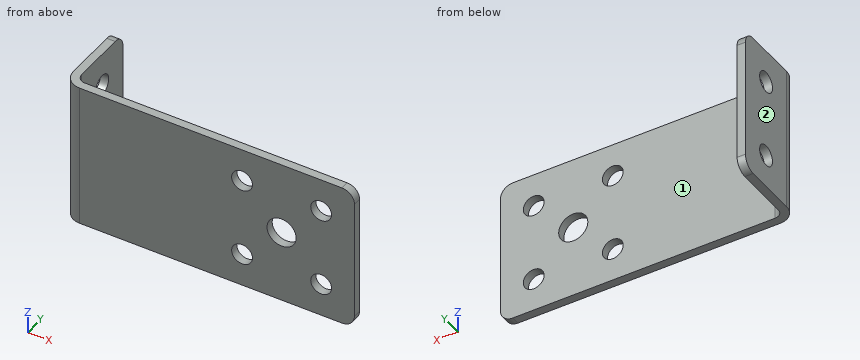
from build123d import *

# Parameters (mm, degrees)
SKETCH1_W                    = 70
SKETCH1_H                    = 35
BASE_FLANGE1_DEPTH           = 2
EDGE_FLANGE1_STRIP_W         = 12
EDGE_FLANGE1_STRIP_H         = 2
EDGE_FLANGE1_STRIP_CUT_DEPTH = 35
EDGE_FLANGE1_DEPTH           = 35
F_5_0MM_DOWEL_HOLE1_D        = 5
F_5_0MM_DOWEL_HOLE2_D        = 7
F_5_0MM_DOWEL_HOLE3_D        = 5
FILLET1_R                    = 3


# Sheet-metal steps are written as plain solids
with BuildPart() as part:
    # Sketch1 → Base-Flange1 (new body)
    with BuildSketch(Plane(origin=(0, 0, 0), x_dir=(1, 0, 0), z_dir=(0, 1, 0))):
        Rectangle(SKETCH1_W, SKETCH1_H)
    extrude(amount=BASE_FLANGE1_DEPTH)

    # Edge-Flange1 strip (across the edge) → Edge-Flange1 strip cut (cut)
    with BuildSketch(Plane(origin=(-35, 2, -17.5), x_dir=(1, 0, 0), z_dir=(0, 0, 1))):
        with Locations((-2, -1)):
            Rectangle(EDGE_FLANGE1_STRIP_W, EDGE_FLANGE1_STRIP_H)
    extrude(amount=EDGE_FLANGE1_STRIP_CUT_DEPTH, mode=Mode.SUBTRACT)

    # Edge-Flange1 section (across the edge) → Edge-Flange1 (add)
    with BuildSketch(Plane(origin=(-35, 2, -17.5), x_dir=(1, 0, 0), z_dir=(0, 0, 1))):
        with BuildLine():
            Line((0, 2), (0, 18))
            Line((0, 18), (2, 18))
            Line((2, 18), (2, 2))
            ThreePointArc((2, 2), (2.585786438, 0.585786438), (4, 0))
            Line((4, 0), (4, -2))
            ThreePointArc((4, -2), (1.171572875, -0.828427125), (0, 2))
        make_face()
    extrude(amount=EDGE_FLANGE1_DEPTH)

    # Ø5.0mm Dowel Hole1 (through all)
    with Locations(Plane(origin=(0, 2, 0), x_dir=(1, 0, 0), z_dir=(0, 1, 0))):
        with Locations((8, 9.5), (27, 9.5), (27, -9.5), (8, -9.5)):
            Hole(F_5_0MM_DOWEL_HOLE1_D / 2)

    # Ø5.0mm Dowel Hole2 (through all)
    with Locations(Plane(origin=(0, 2, 0), x_dir=(1, 0, 0), z_dir=(0, 1, 0))):
        with Locations((17.5, 0)):
            Hole(F_5_0MM_DOWEL_HOLE2_D / 2)

    # Ø5.0mm Dowel Hole3 (through all)
    with Locations(Plane(origin=(-33, 0, 0), x_dir=(0, 0, -1), z_dir=(1, 0, 0))):
        with Locations((-9.5, 12), (9.5, 12)):
            Hole(F_5_0MM_DOWEL_HOLE3_D / 2)

    # Fillet1
    fillet1_edges = [part.edges().sort_by_distance(p)[0] for p in [
        (-34, 20, -17.5),
        (-34, 20, 17.5),
        (35, 1, -17.5),
        (35, 1, 17.5),
    ]]
    fillet(fillet1_edges, radius=FILLET1_R)


solid = part.part
Build history of the part. All positions in model axes, mm. Face numbers are marked on the shaded views. A direction names the side the tool comes from. Coordinates: 2 decimals unless noted, no trailing zeros. Order: outer loops, then holes, each group sorted by start corner. A loop starts at its lowest first (then second) coordinate and runs counter-clockwise, first axis right, second up. Notation, with made-up numbers: (34.25, -35) -> (70.25, -35) arc R27 ccw to (70.25, -13) -> close; hole circle Ø1 at (37, -25.75). An arc over 180 degrees is marked (long way). One line per item, written item: value.
(1) Probe line 1 (Z direction, x = 27, y = 1.5); line 2 (X direction, y = 0.95, z = 9.5); line 3 (X direction, y = 1.2, z = -9.5). List the from-to ranges inside material, lowest first. Write a range as [from, to].
Checked values:
line 1: [-17.5, -12], [-7, 7], [12, 17.5]
line 2: [-33.59, 5.5], [10.5, 24.5], [29.5, 35]
line 3: [-33.86, 5.5], [10.5, 24.5], [29.5, 35]
(2) Slice it at C-C, the plane y = 12. List the corners of the cut face in (x, z), plus the area to 3 significant figures.
Checked values:
outline: (-35, -17.5) -> (-33, -17.5) -> (-33, -12) -> (-35, -12) -> close; (-35, -7) -> (-33, -7) -> (-33, 7) -> (-35, 7) -> close; (-35, 12) -> (-33, 12) -> (-33, 17.5) -> (-35, 17.5) -> close
area: 50.0 mm2
(3) Slice it at A-A, the plane x = 17.5. List the corners of the cut face in (y, z), plus the area to 3 significant figures.
Checked values:
outline: (0, -17.5) -> (2, -17.5) -> (2, -3.5) -> (0, -3.5) -> close; (0, 3.5) -> (2, 3.5) -> (2, 17.5) -> (0, 17.5) -> close
area: 56.0 mm2
(4) Slice it at D-D, the plane x = 8. List the corners of the cut face in (y, z), plus the area to 3 significant figures.
Checked values:
outline: (0, -17.5) -> (2, -17.5) -> (2, -12) -> (0, -12) -> close; (0, -7) -> (2, -7) -> (2, 7) -> (0, 7) -> close; (0, 12) -> (2, 12) -> (2, 17.5) -> (0, 17.5) -> close
area: 50.0 mm2
(5) Slice it at B-B, the plane z = 9.5. List the corners of the cut face in (x, y), plus the area to 3 significant figures.
Checked values:
outline: (-35, 4) arc R4 ccw to (-31, 0) -> (5.5, 0) -> (5.5, 2) -> (-31, 2) arc R2 cw to (-33, 4) -> (-33, 9.5) -> (-35, 9.5) -> close; (-35, 14.5) -> (-33, 14.5) -> (-33, 20) -> (-35, 20) -> close; (10.5, 0) -> (24.5, 0) -> (24.5, 2) -> (10.5, 2) -> close; (29.5, 0) -> (35, 0) -> (35, 2) -> (29.5, 2) -> close
area: 143 mm2
(6) Drop flat-ended pins along their axis: pin 1 Ø4 at (x, z) = (27, 9.5) entering from -Y; pin 2 Ø5 at (y, z) = (11.5, 0) entering from +X; pin 3 Ø1.5 at (x, z) = (9.5, -7.5) entering from +Y. Give the stop position or say it passes through.
Checked values:
pin 1: through
pin 2: x = -33
pin 3: y = 2
(7) Tool access for the marked faces 1 and 2: list every direction of +Z, -Z, +X, -X, +Y, -Y with a clear straight run to the whole face (end or side of a thin tool).
Checked values:
face 1: +Z, -Z, +X, +Y
face 2: +Z, -Z, -X, +Y, -Y
